Here's how the part is built. I have some questions about the finished solid (model axes, mm). Give positions to 0.01 mm unless a question says otherwise; leave off trailing zeros. Order: outer loops, then holes, each group sorted by start corner. A loop starts at its lowest first (then second) coordinate and runs counter-clockwise, first axis right, second up.
from build123d import *

# Parameters (mm, degrees)
BOSS_EXTRUDE1_DEPTH            = 1
SKETCH2_R                      = 1.65
SKETCH2_R_2                    = 0.85
CUT_EXTRUDE1_DEPTH             = 2
CHAMFER1_SIZE                  = 0.15
CHAMFER2_SIZE                  = 0.3
F_0_9_0_9_DIAMETER_HOLE1_D     = 0.9
F_0_9_0_9_DIAMETER_HOLE1_DEPTH = 1


with BuildPart() as part:
    # Sketch1 → Boss-Extrude1 (new body)
    with BuildSketch(Plane.XY):
        with BuildLine():
            Line((0.267857143, 2.988018164), (11.378571429, 1.99201211))
            ThreePointArc((11.378571429, 1.99201211), (13.2, 0), (11.378571429, -1.99201211))
            Line((11.378571429, -1.99201211), (0.267857143, -2.988018164))
            ThreePointArc((0.267857143, -2.988018164), (-3, 0), (0.267857143, 2.988018164))
        make_face()
    extrude(amount=-BOSS_EXTRUDE1_DEPTH)

    # Sketch2 → Cut-Extrude1 (cut, through all)
    with BuildSketch(Plane.XY):
        Circle(SKETCH2_R)
        with Locations((11.2, 0)):
            Circle(SKETCH2_R_2)
    extrude(amount=-CUT_EXTRUDE1_DEPTH, mode=Mode.SUBTRACT)

    # Chamfer1
    chamfer1_edges = [part.edges().sort_by_distance(p)[0] for p in [
        (-1.65, 0, 0),
        (10.35, 0, 0),
    ]]
    chamfer(chamfer1_edges, length=CHAMFER1_SIZE)

    # Chamfer2
    chamfer2_edges = [part.edges().sort_by_distance(p)[0] for p in [
        (-1.65, 0, -1),
    ]]
    chamfer(chamfer2_edges, length=CHAMFER2_SIZE)

    # Ø0.9 (0.9) Diameter Hole1
    with Locations(Plane.XY):
        with Locations((2.9, 0), (2.511473671, 1.45), (2.511473671, -1.45)):
            Hole(F_0_9_0_9_DIAMETER_HOLE1_D / 2, depth=F_0_9_0_9_DIAMETER_HOLE1_DEPTH)


solid = part.part
Q1. I need wall thicknesses on L1, parallel to Y at x = 2.75, z = -0.6; L2, parallel to Y at x = 0, z = -0.35; L3, parallel to Y at x = 11.25, z = -0.75. Which ranges of each line are inside material? Lowest first, please.
Filled sheet:
L1: y = -2.77 to -1.83, -1.07 to -0.42, 0.42 to 1.07, 1.83 to 2.77
L2: y = -3 to -1.65, 1.65 to 3
L3: y = -2 to -0.85, 0.85 to 2
Q2. If we section it at C-C on z = -0.85: List the corners of the cut face in (x, y) for me.
Filled sheet:
outline: (0.27, -2.99) - (11.38, -1.99) arc R2 ccw to (11.38, 1.99) - (0.27, 2.99) arc R3 ccw (long way) to start; hole circle Ø3.6 at (0, 0); hole circle Ø0.9 at (2.51, -1.45); hole circle Ø0.9 at (2.51, 1.45); hole circle Ø0.9 at (2.9, 0); hole circle Ø1.7 at (11.2, 0)
Q3. Thinking about a two-plate mould opening in X: for faces 1 (the face through (11.985, -0.326, -0.569)), 2 (the face through (13.2, 0, -0.5)), 3 (the face through (5, 0, 0)), which applies, released by +X, released by -X, zero draft, split by the parting line, or undercut?
Filled sheet:
face 1: undercut
face 2: released by +X
face 3: zero draft
Q4. If we section it at D-D on y = -1.3: Give the number of separate pieces and of enclosed holes in the cut face, plus the area to 3 significant figures.
Filled sheet:
separate pieces: 3
enclosed holes: 0
area: 12.4 mm2
Q5. If we section it at B-B on y = 0: List the corners of the cut face in (x, z) for me.
Filled sheet:
outline: (-3, -1) - (-1.95, -1) - (-1.65, -0.7) - (-1.65, -0.15) - (-1.8, 0) - (-3, 0) - close; (1.65, -0.7) - (1.95, -1) - (2.45, -1) - (2.45, 0) - (1.8, 0) - (1.65, -0.15) - close; (3.35, -1) - (10.35, -1) - (10.35, -0.15) - (10.2, 0) - (3.35, 0) - close; (12.05, -1) - (13.2, -1) - (13.2, 0) - (12.2, 0) - (12.05, -0.15) - close
Q6. I'm going to push a flat-ended pin straight in: P1, Ø2, axis at x = 8, y = 0, coming from the +Z side. Where does the tip first touch, or does it pass through?
Filled sheet:
P1: stops at z = 0
Q7. If we section it at A-A on x = 0: List the corners of the cut face in (y, z) for me, plus the area to 3 significant figures.
Filled sheet:
outline: (-3, -1) - (-1.95, -1) - (-1.65, -0.7) - (-1.65, -0.15) - (-1.8, 0) - (-3, 0) - close; (1.65, -0.7) - (1.95, -1) - (3, -1) - (3, 0) - (1.8, 0) - (1.65, -0.15) - close
area: 2.59 mm2
